Design review of the part built by this model. Coordinates are the model's own, in mm. Face numbers are marked on the shaded views. A direction names the side the tool comes from. Coordinates: 2 decimals unless noted, no trailing zeros. Order: outer loops, then holes, each group sorted by start corner. A loop starts at its lowest first (then second) coordinate and runs counter-clockwise, first axis right, second up. Notation, with made-up numbers: (73.5, 55.5) - (118.5, 55.5) arc R37 ccw to (118.5, 91.5) - close; hole circle Ø1 at (-16.75, 24.25). An arc over 180 degrees is marked (long way). Write item = value, one per line. Start each with the question number.
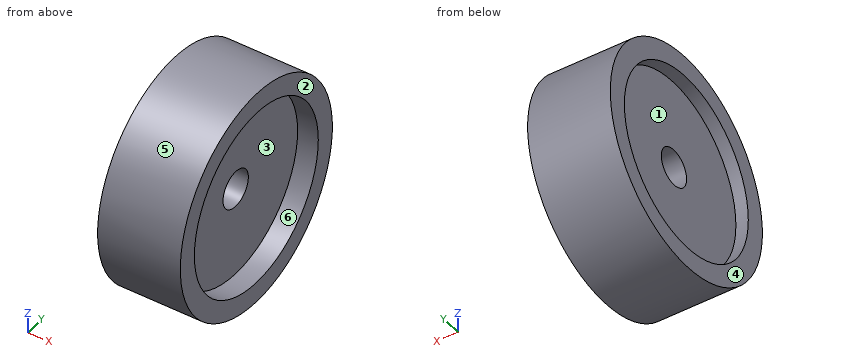
```python
from build123d import *

# Parameters (mm, degrees)
ESQUISSE1_R             = 27
ESQUISSE1_R_2           = 4.5
EXTRUSION1_DEPTH        = 20
ESQUISSE2_R             = 22
ENL_V_MAT_EXTRU_1_DEPTH = 3
ESQUISSE3_R             = 22
ENL_V_MAT_EXTRU_2_DEPTH = 5


with BuildPart() as part:
    # Esquisse1 → Extrusion1 (new body)
    with BuildSketch(Plane(origin=(0, 0, 0), x_dir=(0, 0, -1), z_dir=(1, 0, 0))):
        Circle(ESQUISSE1_R)
        Circle(ESQUISSE1_R_2, mode=Mode.SUBTRACT)
    extrude(amount=EXTRUSION1_DEPTH)

    # Esquisse2 → Enlèv. mat.-Extru.1 (cut)
    with BuildSketch(Plane.ZY):
        Circle(ESQUISSE2_R)
    extrude(amount=-ENL_V_MAT_EXTRU_1_DEPTH, mode=Mode.SUBTRACT)

    # Esquisse3 → Enlèv. mat.-Extru.2 (cut)
    with BuildSketch(Plane(origin=(20, 0, 0), x_dir=(0, 0, -1), z_dir=(1, 0, 0))):
        Circle(ESQUISSE3_R)
    extrude(amount=-ENL_V_MAT_EXTRU_2_DEPTH, mode=Mode.SUBTRACT)


solid = part.part
```
Item 1: For the marked faces 1, 2 and 3, list the 3-axis set-ups (+Z, -Z, +X, -X, +Y, -Y) from which the entire face can be reached by the end or side of a thin tool; tool diameter is ignored.
Item 2: Add section D-D on y = 13.5. Give the boundary of the cut face in (x, z).
Item 3: For line 1 (Y direction, x = 1.45, z = 0); line 2 (Y direction, x = 9.5, z = 1.5); line 3 (X direction, y = 19, z = 5.5), list the stretches that pass through material, from the lowest coordinate up.
Item 4: Add section A-A on z = 0. Give the boundary of the cut face in (x, y), plus the area to 3 significant figures.
Item 5: For P1, Ø12, axis at x = 13.5, y = -6.5, coming from the -Z side; P2, Ø2, axis at x = 3, z = -5, coming from the +Y side; P3, Ø1, axis at y = 8.5, z = 2.5, coming from the +X side; P4, Ø8, axis at y = 0, z = 0, coming from the -X side, all flat-tipped, find the tip position at first contact; note any pin that passes through.
Item 6: Mouldability with a two-part tool opening along Y and no side actions: class the marked faces 4, 5 and 6 as +Y half, -Y half, draft (parallel to the pull), parting line (faces both ways), or undercut.
Item 7: Add section C-C on x = 7.5. Give the boundary of the cut face in (y, z).
Worked out:
q1.face_1 = -X
q1.face_2 = +Z, -Z, +X, +Y, -Y
q1.face_3 = +X
q2.outline = (0, -23.38) - (20, -23.38) - (20, -17.37) - (15, -17.37) - (15, 17.37) - (20, 17.37) - (20, 23.38) - (0, 23.38) - (0, 17.37) - (3, 17.37) - (3, -17.37) - (0, -17.37) - close
q3.line_1 = -27 to -22, 22 to 27
q3.line_2 = -26.96 to -4.24, 4.24 to 26.96
q3.line_3 = 3 to 15
q4.outline = (0, -27) - (20, -27) - (20, -22) - (15, -22) - (15, -4.5) - (3, -4.5) - (3, -22) - (0, -22) - close; (0, 22) - (3, 22) - (3, 4.5) - (15, 4.5) - (15, 22) - (20, 22) - (20, 27) - (0, 27) - close
q4.area = 620 mm2
q5.P1 = -27
q5.P2 = 26.7
q5.P3 = 15
q5.P4 = through
q6.face_4 = draft
q6.face_5 = parting line
q6.face_6 = undercut
q7.outline = circle Ø54 at (0, 0); hole circle Ø9 at (0, 0)
